from build123d import *

# Parameters (mm, degrees)
SKETCH_1_W          = 40
SKETCH_1_H          = 20
EXTRUDE_1_DEPTH     = 10
SKETCH_2_W          = 30
SKETCH_2_H          = 15
EXTRUDE_2_DEPTH     = 6
SKETCH_3_W          = 4
SKETCH_3_H          = 10
CUT_EXTRUDE_1_DEPTH = 40


with BuildPart() as part:
    # 草图1 → 凸台-拉伸1 (new body)
    with BuildSketch(Plane.XY):
        Rectangle(SKETCH_1_W, SKETCH_1_H)
    extrude(amount=EXTRUDE_1_DEPTH)

    # 草图2 → 凸台-拉伸2 (add)
    with BuildSketch(Plane.XY.offset(10)):
        Rectangle(SKETCH_2_W, SKETCH_2_H)
    extrude(amount=EXTRUDE_2_DEPTH)

    # 草图3 → 切除-拉伸1 (cut)
    with BuildSketch(Plane(origin=(15, 0, 0), x_dir=(0, 0, -1), z_dir=(1, 0, 0))):
        with Locations((-12, 0)):
            Rectangle(SKETCH_3_W, SKETCH_3_H)
    extrude(amount=-CUT_EXTRUDE_1_DEPTH, mode=Mode.SUBTRACT)


solid = part.part
Read the model definition and answer for the solid it produces. Units are mm, in the model's axes. A direction names the side the tool comes from. Give positions to 0.01 mm unless a question says otherwise; leave off trailing zeros. Write each loop counter-clockwise with the first axis right and the second up, starting at its lowest first coordinate (ties: lowest second). Pieces come first, ordered by that corner, then holes. Notation, with made-up numbers: M -23.75,85.25 L 16.25,85.25 A15 ccw 16.25,113.25 Z; hole C 70.25,54 d6. An arc over 180 degrees is marked long. One line per item, written item: value. Start each with the question number.
(1) A tool of negligible diameter and unlimited length cuts with its end or side. For faces 1 (the flat face through (15, -0.1, 14.3)), 2 (the flat face through (0, -7.5, 13)), 3 (the flat face through (0, 0, 14)), from which of +Z, -Z, +X, -X, +Y, -Y can it reach the whole face along a straight path? Write none if from no direction.
(2) Find section C-C (x = 14). Determine the outline of the cut face in (y, z).
(3) Find section D-D (y = -6). Determine the outline of the cut face in (x, z), plus the area to 3 significant figures.
(4) Flat-ended cylindrical pins translate along their axes: pin 1 Ø3 at (x, z) = (14, 10.5) entering from -Y; pin 2 Ø4.5 at (x, z) = (1, 13) entering from +Y; pin 3 Ø3 at (y, z) = (-3, 13) entering from -X; pin 4 Ø3 at (y, z) = (-2.5, 14.5) entering from +X. Find the tip coordinate at first contact, or state that the pin passes through.
(5) Find section A-A (y = 1.75). Determine the outline of the cut face in (x, z).
(6) Find section B-B (z = 13.5). Determine the outline of the cut face in (x, y), plus the area to 3 significant figures.
(7) Find the intervals of material crossed by line 1 (Z direction, x = -6.5, y = -4.5); line 2 (Y direction, x = -4, z = 10.75); line 3 (X direction, y = 2.25, z = 15), in increasing order.
(8) Determine the mould class of faces 4 (the flat face through (0, 7.5, 13)), 5 (the flat face through (0, 0, 10)), 6 (the flat face through (-15, -0.1, 14.3)) for opening direction Y: pulls with the +Y half, pulls with the -Y half, needs draft (parallel to the pull), parting line crosses it, or undercut.
Results below:
1. face 1: +Z, +X, +Y, -Y
1. face 2: +Z, +X, -X, -Y
1. face 3: +X, -X
2. outline: M -10,0 L 10,0 L 10,10 L 7.5,10 L 7.5,16 L -7.5,16 L -7.5,10 L -10,10 Z; hole M -5,10 L 5,10 L 5,14 L -5,14 Z
3. outline: M -20,0 L 20,0 L 20,10 L 15,10 L 15,16 L -15,16 L -15,10 L -20,10 Z
3. area: 580 mm^2
4. pin 1: stops at y = -10
4. pin 2: stops at y = 7.5
4. pin 3: stops at x = -15
4. pin 4: stops at x = 15
5. outline: M -20,0 L 20,0 L 20,10 L -20,10 Z; M -15,14 L 15,14 L 15,16 L -15,16 Z
6. outline: M -15,-7.5 L 15,-7.5 L 15,-5 L -15,-5 Z; M -15,5 L 15,5 L 15,7.5 L -15,7.5 Z
6. area: 150 mm^2
7. line 1: z = 0 to 10, 14 to 16
7. line 2: y = -7.5 to -5, 5 to 7.5
7. line 3: x = -15 to 15
8. face 4: pulls with the +Y half
8. face 5: undercut
8. face 6: needs draft
